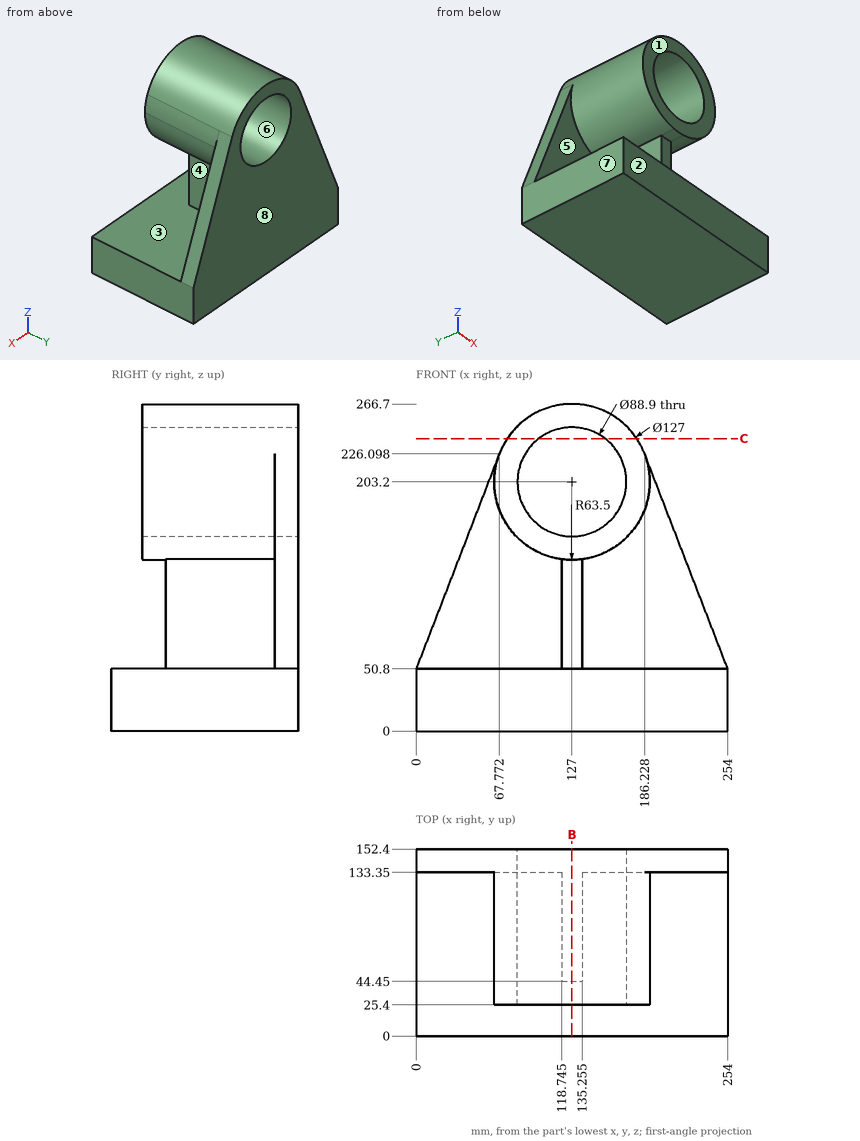
Verification items for this drawing (mm, ordinates from the low corner). A direction names the side the tool comes from. Round coordinates to 2 decimals unless told otherwise and drop trailing zeros. Loops run counter-clockwise (first coordinate to the right, second up) from the corner with the lowest first, then second, coordinate; pieces in that order, holes last. Notation, with made-up numbers: (-2.5, 80) -> (11.5, 80) arc R31 cw to (11.5, 115) -> close; hole circle Ø6 at (-35, 44.5). An arc over 180 degrees is marked (long way). Write item = value, one per line. Start each with the question number.
1) Thickness scan on probe 1 along Z at (x, y) = (127, 79.5); probe 2 along X at (y, z) = (79, 203); probe 3 along Z at (x, y) = (183, 19). Record the ranges inside material, lowest first.
2) Sectioned sample at C-C, the plane z = 238.5. Record the cut outline in (x, y), plus the area to 3 significant figures.
3) Set-up check for the marked faces 1, 2, 3, 4 and 5: record each of +Z, -Z, +X, -X, +Y, -Y from which the full face is reachable in a straight line by a thin tool's end or side.
4) Sectioned sample at B-B, the plane x = 127. Record the cut outline in (y, z).
5) Release check for a two-part mould opening along X. For the marked faces 6, 7 and 8 record: released by +X, released by -X, zero draft, split by the parting line, or undercut.
6) Gauge pin test, flat ends, axial feed: pin 1 Ø10 at (x, y) = (42, 70) entering from +Z; pin 2 Ø13 at (x, z) = (129, 76) entering from -Y; pin 3 Ø4 at (x, y) = (67.5, 44.5) entering from +Z (1 decimal). Record the tip position at first contact, or that the pin passes through.
Results are:
q1.probe_1 = 0 to 158.75, 247.65 to 266.7
q1.probe_2 = 63.5 to 82.55, 171.45 to 190.5
q1.probe_3 = 0 to 50.8
q2.outline = (74.22, 25.4) -> (99.99, 25.4) -> (99.99, 152.4) -> (74.22, 152.4) -> close; (154.01, 25.4) -> (179.78, 25.4) -> (179.78, 152.4) -> (154.01, 152.4) -> close
q2.area = 6,550 mm^2
q3.face_1 = +Z, +X, -X, -Y
q3.face_2 = +Z, -Z, +X, -X, -Y
q3.face_3 = -Y
q3.face_4 = +X, -Y
q3.face_5 = -X, -Y
q4.outline = (0, 0) -> (152.4, 0) -> (152.4, 158.75) -> (25.4, 158.75) -> (25.4, 139.7) -> (44.45, 139.7) -> (44.45, 50.8) -> (0, 50.8) -> close; (25.4, 247.65) -> (152.4, 247.65) -> (152.4, 266.7) -> (25.4, 266.7) -> close
q5.face_6 = undercut
q5.face_7 = released by -X
q5.face_8 = zero draft
q6.pin_1 = 50.8
q6.pin_2 = 44.45
q6.pin_3 = 230.1
